Autodesk Inventor part; units mm, degrees
ref_plane "YZ Plane" through (0, 0, 0) normal (1, 0, 0) x (0, 1, 0)
ref_plane "XZ Plane" through (0, 0, 0) normal (0, 1, 0) x (-1, 0, 0)
ref_plane "XY Plane" through (0, 0, 0) normal (0, 0, 1) x (1, 0, 0)
sketch "Sketch1" plane through (0, 0, 0) normal (0, 0, 1) x (1, 0, 0)
  line L0 (0, 0) -> (-69.85, 0)
  line L1 (-69.85, 0) -> (-69.85, 57.15)
  line L2 (-69.85, 57.15) -> (0, 57.15)
  line L3 (0, 57.15) -> (0, 0)
  dimension "d0" = 69.85
  dimension "d1" = 57.15
extrude "Extrusion1" add sketch "Sketch1" along normal blind 3.175
sketch "Sketch2" plane through (0, 0, 3.175) normal (0, 0, 1) x (1, 0, 0)
  line L0 (-69.85, 57.15) -> (-69.85, 0) construction
  line L1 (-69.85, 0) -> (0, 0) construction
  line L2 (-69.85, 57.15) -> (0, 0) construction
  circle A0 centre (-34.925, 28.575) radius 22.225
  dimension "d4" = 44.45
extrude "Extrusion2" add sketch "Sketch2" along normal blind 3.175
sketch "Sketch3" plane through (0, 0, 3.175) normal (0, 0, 1) x (1, 0, 0)
  circle A0 centre (-34.925, 28.575) radius 22.225 construction
  circle A1 centre (-34.925, 28.575) radius 31.75 construction
  line L0 (-34.925, 28.575) -> (-12.4744, 6.1244) construction
  line L1 (-34.925, 28.575) -> (-3.175, 28.575) construction
  circle A2 centre (-12.4744, 6.1244) radius 3.1
  circle A3 centre (-12.4744, 51.0256) radius 3.1
  circle A4 centre (-57.3756, 51.0256) radius 3.1
  circle A5 centre (-57.3756, 6.1244) radius 3.1
  point P0 (0, 0)
  dimension "d7" = 63.5
  dimension "d8" = 45
  dimension "d9" = 6.2
  dimension "d12" = 360
extrude "Extrusion3" cut sketch "Sketch3" against normal blind 3.175
properties part number "endcap1" material "Aluminum 6061"
The model under review builds one solid part; all positions refer to its coordinate system, in mm. A direction names the side the tool comes from. Give positions to 0.01 mm unless a question says otherwise; leave off trailing zeros. Write each loop counter-clockwise with the first axis right and the second up, starting at its lowest first coordinate (ties: lowest second). Pieces come first, ordered by that corner, then holes.
(1) Tool access review of faces 1 (the flat face through (-35, 57.15, 2)), 2 (the flat face through (-59, 29, 3.175)): name each direction out of +Z, -Z, +X, -X, +Y, -Y from which nothing blocks a thin tool from reaching the whole face with its end or side.
(2) Consider section B-B, the plane y = 4.5. Give the boundary of the cut face in (x, z) (3 decimals).
(3) The part is to be moulded in two halves that separate along Y. For faces 3 (the flat face through (-69.85, 28, 2)), 4 (the flat face through (-34, 0, 2)), 5 (the cylindrical face through (-57.78, 54.1, 1.61)), 6 (the cylindrical face through (-10.81, 8.74, 1.61)), say which applies: released by +Y, released by -Y, zero draft, split by the parting line, or undercut.
(4) For P1, Ø5, axis at x = -57.38, y = 51.03, coming from the +Z side; P2, Ø10, axis at x = -12.47, y = 51.03, coming from the +Z side (3 decimals); P3, Ø2, axis at x = -33.5, z = 5, coming from the +Y side, all flat-tipped, find the tip position at first contact; note any pin that passes through.
(5) Consider section A-A, the plane x = -10.5. Give the boundary of the cut face in (y, z) (3 decimals).
(6) Consider section C-C, the plane z = 1.5. Give the boundary of the cut face in (x, y).
(7) To check wall thickness, follow L1, parallel to X at y = 6, z = 0.5; L2, parallel to Z at x = -6, y = 30 (3 decimals); L3, parallel to Y at x = -24.5, z = 5.5. State the ranges of each line that lie inside material, in increasing order.
(8) Consider section D-D, the plane x = -28. Give the boundary of the cut face in (y, z) (3 decimals), and give its area (3 significant figures).
Returned:
1. face 1: +Z, -Z, +X, -X, +Y
1. face 2: +Z
2. outline: (-69.85, 0) - (-60.016, 0) - (-60.016, 3.175) - (-69.85, 3.175) - close; (-54.735, 0) - (-15.115, 0) - (-15.115, 3.175) - (-54.735, 3.175) - close; (-9.834, 0) - (0, 0) - (0, 3.175) - (-9.834, 3.175) - close
3. face 3: zero draft
3. face 4: released by -Y
3. face 5: undercut
3. face 6: undercut
4. P1: passes through
4. P2: stops at z = 3.175
4. P3: stops at y = 50.8
5. outline: (0, 0) - (3.734, 0) - (3.734, 3.175) - (0, 3.175) - close; (8.514, 0) - (48.636, 0) - (48.636, 3.175) - (8.514, 3.175) - close; (53.416, 0) - (57.15, 0) - (57.15, 3.175) - (53.416, 3.175) - close
6. outline: (-69.85, 0) - (0, 0) - (0, 57.15) - (-69.85, 57.15) - close; hole circle Ø6.2 at (-57.38, 6.12); hole circle Ø6.2 at (-57.38, 51.03); hole circle Ø6.2 at (-12.47, 6.12); hole circle Ø6.2 at (-12.47, 51.03)
7. L1: x = -69.85 to -60.47, -54.28 to -15.57, -9.38 to 0
7. L2: z = 0 to 3.175
7. L3: y = 8.95 to 48.2
8. outline: (0, 0) - (57.15, 0) - (57.15, 3.175) - (49.694, 3.175) - (49.694, 6.35) - (7.456, 6.35) - (7.456, 3.175) - (0, 3.175) - close
8. area: 316 mm2
